Read the model definition and answer for the solid it produces. Units are mm, in the model's axes. Face numbers are marked on the shaded views. A direction names the side the tool comes from. Give positions to 0.01 mm unless a question says otherwise; leave off trailing zeros. Order: outer loops, then holes, each group sorted by start corner. A loop starts at its lowest first (then second) coordinate and runs counter-clockwise, first axis right, second up. Notation, with made-up numbers: (9.25, 79.5) - (57.25, 79.5) arc R16 ccw to (57.25, 99.5) - close; hole circle Ø8 at (-38.75, -23). An arc over 180 degrees is marked (long way). Return JSON: item names as keys, results as strings.
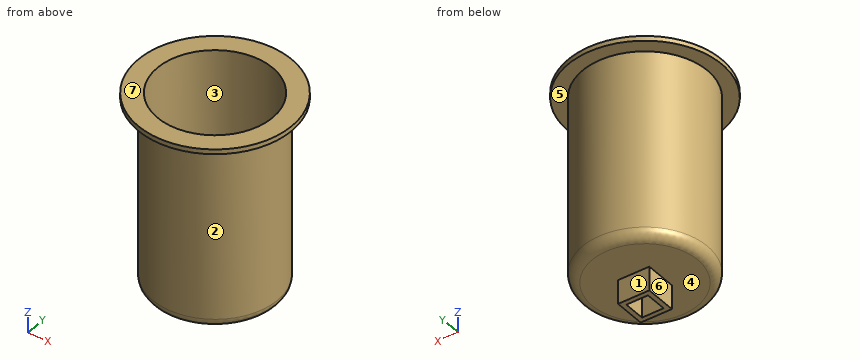
Autodesk Inventor part; units mm, degrees
ref_plane "YZ Plane" through (0, 0, 0) normal (1, 0, 0) x (0, 1, 0)
ref_plane "XZ Plane" through (0, 0, 0) normal (0, 1, 0) x (-1, 0, 0)
ref_plane "XY Plane" through (0, 0, 0) normal (0, 0, 1) x (1, 0, 0)
sketch "Эскиз1" plane through (0, 0, 0) normal (0, 0, 1) x (1, 0, 0)
  circle A0 centre (0, 0) radius 13
  circle A1 centre (0, 0) radius 12
  dimension "d0" = 26
  dimension "d1" = 24
extrude "Выдавливание1" add sketch "Эскиз1" along normal blind 38
sketch "Эскиз2" plane through (0, 0, 38) normal (0, 0, 1) x (1, 0, 0)
  circle A0 centre (0, 0) radius 16
  circle A1 centre (0, 0) radius 12
  dimension "d4" = 32
  dimension "d5" = 24
extrude "Выдавливание2" add sketch "Эскиз2" along normal blind 1
sketch "Эскиз3" plane through (0, 0, 0) normal (0, 0, -1) x (-1, 0, 0)
  circle A0 centre (0, 0) radius 13
extrude "Выдавливание3" add sketch "Эскиз3" along normal blind 1
fillet "Сопряжение1" radius 2 1 edges at (-12, 0, 0)
fillet "Сопряжение2" radius 2 1 edges at (13, 0, -1)
sketch "Эскиз4" plane through (0, 0, -1) normal (0, 0, -1) x (-1, 0, 0)
  line L0 (-2.25, -2.25) -> (2.25, -2.25)
  line L1 (2.25, -2.25) -> (2.25, 2.25)
  line L2 (2.25, 2.25) -> (-2.25, 2.25)
  line L3 (-2.25, 2.25) -> (-2.25, -2.25)
  line L4 (22.4, 0) -> (-22.4, 0)
  line L5 (0, -22.4) -> (0, 22.4)
  point P0 (0, 0)
  dimension "d12" = 4.5
  dimension "d13" = 4.5
extrude "Выдавливание4" cut sketch "Эскиз4" against normal blind 1
sketch "Эскиз5" plane through (0, 0, -1) normal (0, 0, -1) x (-1, 0, 0)
  line L0 (-2.25, 2.25) -> (2.25, 2.25)
  line L1 (-2.25, -2.25) -> (-2.25, 2.25)
  line L2 (2.25, -2.25) -> (-2.25, -2.25)
  line L3 (2.25, 2.25) -> (2.25, -2.25)
  line L4 (-3.25, -3.25) -> (3.25, -3.25)
  line L5 (3.25, -3.25) -> (3.25, 3.25)
  line L6 (3.25, 3.25) -> (-3.25, 3.25)
  line L7 (-3.25, 3.25) -> (-3.25, -3.25)
  point P0 (0, 0)
  dimension "d16" = 1
  dimension "d17" = 1
  dimension "d18" = 1
  dimension "d19" = 1
extrude "Выдавливание5" add sketch "Эскиз5" along normal blind 5
properties part number "насадка для катпака"
Q1. A cutting plane is placed at B-B (z = 22.5). Write down the section's boundary in (x, y).
Values:
{"outline": "circle Ø26 at (0, 0); hole circle Ø24 at (0, 0)"}
Q2. Given pin 1 (2 mm diameter, centred on x = 0.5, z = -3.5, fed in from +Y); pin 2 (1.3 mm diameter, centred on y = 0.5, z = -3.5, fed in from -X); pin 3 (1.3 mm diameter, centred on x = 1, z = -3, fed in from -Y), each flat-ended and moving along its own axis, determine where each tip first touches the part or whether it passes through.
Values:
{"pin 1": "stops at y = 3.25", "pin 2": "stops at x = -3.25", "pin 3": "stops at y = -3.25"}
Q3. A cutting plane is placed at A-A (z = -3). Write down the section's boundary in (x, y), and give its area (3 significant figures).
Values:
{"outline": "(-3.25, -3.25) - (3.25, -3.25) - (3.25, 3.25) - (-3.25, 3.25) - close; hole (-2.25, -2.25) - (2.25, -2.25) - (2.25, 2.25) - (-2.25, 2.25) - close", "area": "22.0 mm²"}
Q4. A cutting plane is placed at C-C (y = 14). Write down the section's boundary in (x, z).
Values:
{"outline": "(-7.75, 38) - (7.75, 38) - (7.75, 39) - (-7.75, 39) - close"}
Q5. Consider L1, parallel to Y at x = 0, z = 18; L2, parallel to Z at x = -4, y = 6.5; L3, parallel to Z at x = -12.5, y = 6.5. Determine where each line is inside the solid, lowest interval first.
Values:
{"L1": "y = -13 to -12, 12 to 13", "L2": "z = -1 to 0", "L3": "z = 38 to 39"}
Q6. For the marked faces 5, 6 and 7, determine the directions among +Z, -Z, +X, -X, +Y, -Y from which every point of the face is accessible in a straight line to the end or side of a thin tool.
Values:
{"face 5": "-Z", "face 6": "-Z, -X, +Y, -Y", "face 7": "+Z, +X, -X, +Y, -Y"}
Q7. Determine the mould class of the marked faces 1, 2, 3 and 4 for opening direction Y: released by +Y, released by -Y, zero draft, split by the parting line, or undercut.
Values:
{"face 1": "released by +Y", "face 2": "split by the parting line", "face 3": "undercut", "face 4": "zero draft"}
